Design review of the part shown in the three views and the two pictorial views. Dimensions are in mm from the part's minimum x, y and z. A direction names the side the tool comes from. Round coordinates to 2 decimals unless told otherwise and drop trailing zeros. Loops run counter-clockwise (first coordinate to the right, second up) from the corner with the lowest first, then second, coordinate; pieces in that order, holes last. Notation, with made-up numbers: M 50,5.25 L 90,5.25 A20 cw 90,26.25 Z; hole C 4.5,48 d6. An arc over 180 degrees is marked long. Return JSON: item names as keys, results as strings. Group by question number.
Q1. Consider section D-D (x = 1.75). State the section outline as (y, z) points, and give its area (3 significant figures).
Q2. Consider section C-C (x = 17.75). State the section outline as (y, z) points.
Q3. Consider section B-B (z = 36). State the section outline as (x, y) points, and give its area (3 significant figures).
Q4. Consider section A-A (y = 12.75). State the section outline as (x, z) points.
Q5. To check wall thickness, follow line 1 along Z through (x, y) = (14.5, 19.25); line 2 along Y through (x, z) = (11.5, 4); line 3 along Y through (x, z) = (23.75, 55). State the ranges of each line that lie inside material, in increasing order.
Q6. For the marked faces 1 and 2, list the 3-axis set-ups (+Z, -Z, +X, -X, +Y, -Y) from which the entire face can be reached by the end or side of a thin tool; tool diameter is ignored.
Q7. Clearance check with flat-ended pins moving along their axes: pin 1 Ø1 at (x, z) = (7, 31) entering from -Y; pin 2 Ø1.8 at (x, z) = (12, 5) entering from -Y; pin 3 Ø4 at (x, y) = (11, 22.5) entering from -Z; pin 4 Ø3 at (y, z) = (13, 4.5) entering from -X. State where each tip first meets the part, or that it passes through.
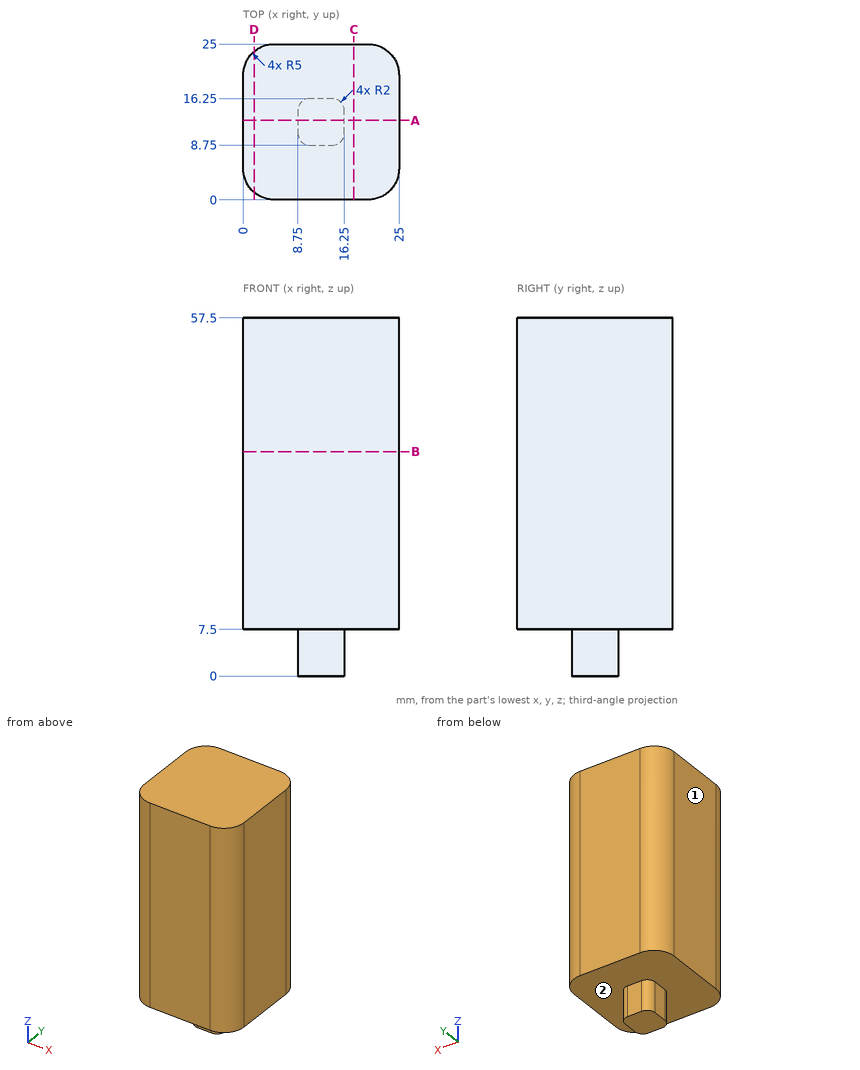
Values:
{
 "1": {"outline": "M 1.2,7.5 L 23.8,7.5 L 23.8,57.5 L 1.2,57.5 Z", "area": "1,130 mm2"},
 "2": {"outline": "M 0,7.5 L 25,7.5 L 25,57.5 L 0,57.5 Z"},
 "3": {"outline": "M 0,5 A5 ccw 5,0 L 20,0 A5 ccw 25,5 L 25,20 A5 ccw 20,25 L 5,25 A5 ccw 0,20 Z", "area": "604 mm2"},
 "4": {"outline": "M 0,7.5 L 8.75,7.5 L 8.75,0 L 16.25,0 L 16.25,7.5 L 25,7.5 L 25,57.5 L 0,57.5 Z"},
 "5": {"line 1": "z = 7.5 to 57.5", "line 2": "y = 8.75 to 16.25", "line 3": "y = 1.69 to 23.31"},
 "6": {"face 1": "+Z, -Z, -X, +Y, -Y", "face 2": "-Z"},
 "7": {"pin 1": "stops at y = 0", "pin 2": "stops at y = 8.75", "pin 3": "stops at z = 7.5", "pin 4": "stops at x = 8.75"}
}
